from build123d import *

# Parameters (mm, degrees)
SKETCH001_R   = 3.4
SKETCH001_R_2 = 0.9
PAD_DEPTH     = 2


with BuildPart() as part:
    # Sketch → Revolution (revolve)
    with BuildSketch(Plane.XZ):
        Polygon((0.9, 12.4), (0.9, 0), (17.75, 0), (17.75, 0.1), (16.2, 1.35), (16.2, 2.35), (17.75, 3.6), (17.75, 3.7), (3.4, 3.7), (3.4, 8.7), (17.75, 8.7), (17.75, 8.8), (16.2, 10.05), (16.2, 11.05), (17.75, 12.3), (17.75, 12.4), align=None)
    revolve(axis=Axis((0, 0, 0), (0, 0, 1)))

    # Sketch001 (on Face1 of Revolution) → Pad (new body)
    with BuildSketch(Plane(origin=(0, 0, 12.4), x_dir=(-1, 0, 0), z_dir=(0, 0, 1))):
        Circle(SKETCH001_R)
        Circle(SKETCH001_R_2, mode=Mode.SUBTRACT)
    extrude(amount=PAD_DEPTH)


solid = part.part
Verification items for the finished model (mm, model axes). A direction names the side the tool comes from. Coordinates: 2 decimals unless noted, no trailing zeros. Order: outer loops, then holes, each group sorted by start corner. A loop starts at its lowest first (then second) coordinate and runs counter-clockwise, first axis right, second up.
Item 1: Depth check by flat-ended pin: pin 1 (5 mm diameter, centred on x = -12.5, z = 8.5, fed in from +Y); pin 2 (6 mm diameter, centred on y = 13, z = 2.5, fed in from +X); pin 3 (1 mm diameter, centred on y = 11, z = 4, fed in from -X). Enter the tip coordinate at first touch or a pass-through.
Filled in:
pin 1: stops at y = 14.66
pin 2: stops at x = 14.52
pin 3: stops at x = -14.24
Item 2: Section check A-A, the plane z = 5. Enter the section's corners in (x, y).
Filled in:
outline: circle Ø6.8 at (0, 0); hole circle Ø1.8 at (0, 0)
Item 3: Access from +Z, -Z, +X, -X, +Y, -Y to the whole of each face (thin tool, end or side, straight path). Record for faces 4 (the face through (-1, 1, 14.4)), 5 (the face through (-3.512, -15.815, 10.557)).
Filled in:
face 4: +Z, +X, -X, +Y, -Y
face 5: none
Item 4: Release check for a two-part mould opening along Z. For faces 1 (the face through (-3.512, -15.815, 1.857)), 2 (the face through (0, -4, 0)), 3 (the face through (0.74, 3.32, 13.39)) record: +Z half, -Z half, draft (parallel to the pull), parting line (faces both ways), or undercut.
Filled in:
face 1: undercut
face 2: -Z half
face 3: draft
Item 5: Material ranges on L1, parallel to Y at x = 0, z = 8.25; L2, parallel to Z at x = -3, y = -8; L3, parallel to Z at x = 8, y = 14.5, recorded low to high.
Filled in:
L1: y = -3.4 to -0.9, 0.9 to 3.4
L2: z = 0 to 3.7, 8.7 to 12.4
L3: z = 0 to 1.06, 2.64 to 3.7, 8.7 to 9.76, 11.34 to 12.4
